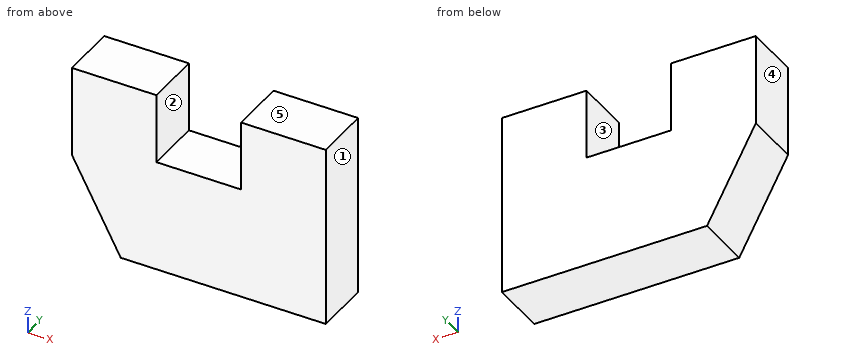
```python
from build123d import *

# Parameters (mm, degrees)
F1_DEPTH = 200
F4_DEPTH = 25
F5_DEPTH = 400


with BuildPart() as f1:
    # F0 (on Front) → F1 (new body)
    with BuildSketch(Plane.XZ):
        Polygon((-1.4871466187, 391.6978864931), (-301.4871466187, 391.6978864931), (-301.4871466187, -258.3021135069), (-190.924435854, -258.3021135069), (-80.4046094418, -258.3021135069), (598.5128533813, -258.3021135069), (598.5128533813, -237.8309071064), (598.5128533813, 391.6978864931), (298.5128533813, 391.6978864931), (298.5128533813, 141.6978864931), (-1.4871466187, 141.6978864931), align=None)
    extrude(amount=F1_DEPTH)

    # F2 (on face) → F4 (cut)
    with BuildSketch(Plane.XZ.offset(200)):
        Polygon((-301.4871466187, 66.6978864931), (-301.4871466187, -258.3021135069), (-128.4365952015, -258.3021135069), align=None)
    extrude(amount=-F4_DEPTH, mode=Mode.SUBTRACT)

    # F5 (cut): a face of the model
    f5_faces = [f1.faces().sort_by_distance(p)[0] for p in [
        (-243.8036294796, -175, -149.9687801736),
    ]]
    extrude(f5_faces, amount=-F5_DEPTH, mode=Mode.SUBTRACT)


solid = f1.part
```
Geometry: final body of the model. Coordinates: model frame, mm. Face numbers are marked on the shaded views. A direction names the side the tool comes from. Give positions to 0.01 mm unless a question says otherwise; leave off trailing zeros. Order: outer loops, then holes, each group sorted by start corner. A loop starts at its lowest first (then second) coordinate and runs counter-clockwise, first axis right, second up. Notation, with made-up numbers: (38.5, -17) -> (63.5, -17) arc R16 cw to (63.5, 8) -> close; hole circle Ø9 at (-29, 71). An arc over 180 degrees is marked (long way). Write each question's results on one line, items separated by ' | '. Start each with the question number.
1) Section B-B (y = -164.5). Return loops of the section in (x, z).
2) Section D-D (z = -169.5). Return loops of the section in (x, y), then the cut area to 3 significant figures.
3) Draft query along X for the marked faces 3, 4 and 5. Return one class per face: pulls with the +X half, pulls with the -X half, needs draft (parallel to the pull), parting line crosses it, or undercut.
4) Set-up query: the marked faces 1 and 2. Return all of +Z, -Z, +X, -X, +Y, -Y with unobstructed straight access to the full face (end or side cutting, diameter ignored); none if empty.
5) First-contact query: pin 1 (1.5 mm diameter, centred on y = -47.5, z = -116, fed in from -X); pin 2 (1.5 mm diameter, centred on x = 142.5, z = -22.5, fed in from +Y). Flat tips, straight axial feed; report the tip coordinate or a pass-through.
6) Line query: line 1 (X direction, y = -182, z = 315.5); line 2 (Z direction, x = 79, y = -189.5); line 3 (Z direction, x = -128.5, y = -111). Output: solid intervals per line, ascending. Write a range as from..to.
7) Section A-A (z = 315.5). Return loops of the section in (x, y).
8) Section C-C (x = 100). Return loops of the section in (y, z), then the cut area to 3 significant figures.
Calculated:
1) outline: (-301.49, 66.7) -> (-128.44, -258.3) -> (598.51, -258.3) -> (598.51, 391.7) -> (298.51, 391.7) -> (298.51, 141.7) -> (-1.49, 141.7) -> (-1.49, 391.7) -> (-301.49, 391.7) -> close
2) outline: (-175.72, -200) -> (598.51, -200) -> (598.51, 0) -> (-175.72, 0) -> close | area: 155,000 mm2
3) face 3: undercut | face 4: pulls with the -X half | face 5: needs draft
4) face 1: +Z, -Z, +X, +Y, -Y | face 2: +Z, +Y, -Y
5) pin 1: x = -204.61 | pin 2: y = 0
6) line 1: -301.49..-1.49, 298.51..598.51 | line 2: -258.3..141.7 | line 3: -258.18..391.7
7) outline: (-301.49, -200) -> (-1.49, -200) -> (-1.49, 0) -> (-301.49, 0) -> close; (298.51, -200) -> (598.51, -200) -> (598.51, 0) -> (298.51, 0) -> close
8) outline: (-200, -258.3) -> (0, -258.3) -> (0, 141.7) -> (-200, 141.7) -> close | area: 80,000 mm2
